```python
from build123d import *

# Parameters (mm, degrees)
F0_W     = 609.6
F0_H     = 88.9
F2_DEPTH = 38.1
F4_DEPTH = 88.901
F5_W     = 38.1
F5_H     = 3.175
F5_W_2   = 533.4
F1_DEPTH = 17.4625


with BuildPart() as f2:
    # F0 (on Top) → F2 (new body)
    with BuildSketch(Plane.XY):
        Rectangle(F0_W, F0_H)
    extrude(amount=F2_DEPTH)

    # F3 (on face) → F4 (cut, through all)
    with BuildSketch(Plane.XZ.offset(44.45)):
        Polygon((-266.7, 0), (-304.8, 38.1), (-304.8, 0), align=None)
        Polygon((304.8, 0), (304.8, 38.1), (266.7, 0), align=None)
    extrude(amount=-F4_DEPTH, mode=Mode.SUBTRACT)

    # F5 (on face) → F1 (cut)
    with BuildSketch(Plane(origin=(0, 0, 0), x_dir=(1, 0, 0), z_dir=(0, 0, -1))):
        with Locations((285.75, 31.75)):
            Rectangle(F5_W, F5_H)
        with Locations((0, 31.75)):
            Rectangle(F5_W_2, F5_H)
        with Locations((-285.75, 31.75)):
            Rectangle(F5_W, F5_H)
    extrude(amount=-F1_DEPTH, mode=Mode.SUBTRACT)


solid = f2.part
```
Here's how the part is built. I have some questions about the finished solid (model axes, mm). A direction names the side the tool comes from. Round coordinates to 2 decimals unless told otherwise and drop trailing zeros. Order: outer loops, then holes, each group sorted by start corner. A loop starts at its lowest first (then second) coordinate and runs counter-clockwise, first axis right, second up. Notation, with made-up numbers: M -3.75,32.5 L 14.25,32.5 A7 cw 14.25,42.5 Z; hole C -3,73 d4. An arc over 180 degrees is marked long. One line per question, with ' | ' between items.
1) I want a section at D-D, the plane z = 31.5. Write out the boundary of the cut face in (x, y).
Working result:
outline: M -298.2,-44.45 L 298.2,-44.45 L 298.2,44.45 L -298.2,44.45 Z
2) For pin 1 Ø8 at (y, z) = (-27.5, 32) entering from +X; pin 2 Ø10 at (x, y) = (-35, 10.5) entering from -Z; pin 3 Ø1 at (x, y) = (59, -31.5) entering from -Z; pin 4 Ø3 at (y, z) = (31.5, 13.5) entering from +X, each with a flat end and sliding along its axis, tell me the tip position at first contact or that it passes through.
Working result:
pin 1: x = 302.7 | pin 2: z = 0 | pin 3: z = 17.46 | pin 4: x = 281.7
3) I need wall thicknesses on line 1 along Y through (x, z) = (-160, 13); line 2 along X through (y, z) = (33, 19); line 3 along X through (y, z) = (-6, 5.5). Which ranges of each line are inside material? Lowest first, please.
Working result:
line 1: -44.45 to -33.34, -30.16 to 44.45 | line 2: -285.7 to 285.7 | line 3: -272.2 to 272.2
4) If we mould it in two halves opening along Y, with no side actions, what happens to faces 3 (the face through (4, -33.338, 9)), 4 (the face through (-4, -44.45, 19)), 5 (the face through (286, -0.6, 19.3))? For each: +Y half, -Y half, draft (parallel to the pull), parting line (faces both ways), or undercut.
Working result:
face 3: undercut | face 4: -Y half | face 5: draft
5) I want a section at B-B, the plane x = -226. Write out the boundary of the cut face in (y, z).
Working result:
outline: M -44.45,0 L -33.34,0 L -33.34,17.46 L -30.16,17.46 L -30.16,0 L 44.45,0 L 44.45,38.1 L -44.45,38.1 Z
6) For faces 1 (the face through (-4, -30.162, 9)), 2 (the face through (-4, -39, 0)), which set-ups out of +Z, -Z, +X, -X, +Y, -Y let a thin tool reach every point of the face, with its end or its side?
Working result:
face 1: -Z, +X, -X | face 2: -Z, +X, -X, +Y, -Y
7) I want a section at A-A, the plane z = 7.5. Write out the boundary of the cut face in (x, y).
Working result:
outline: M -274.2,-44.45 L 274.2,-44.45 L 274.2,-33.34 L -274.2,-33.34 Z; M -274.2,-30.16 L 274.2,-30.16 L 274.2,44.45 L -274.2,44.45 Z
8) I want a section at C-C, the plane y = 39.5. Write out the boundary of the cut face in (x, z).
Working result:
outline: M -304.8,38.1 L -266.7,0 L 266.7,0 L 304.8,38.1 Z
